Here's how the part is built. I have some questions about the finished solid (model axes, mm). A direction names the side the tool comes from. Round coordinates to 2 decimals unless told otherwise and drop trailing zeros. Write each loop counter-clockwise with the first axis right and the second up, starting at its lowest first coordinate (ties: lowest second). Pieces come first, ordered by that corner, then holes. Notation, with made-up numbers: (54, 54) -> (110, 54) arc R9 ccw to (110, 64) -> close; hole circle Ø6 at (-20, -30). An arc over 180 degrees is marked (long way). Answer in a Markdown table with one row per item. Add a question column.
from build123d import *

# Parameters (mm, degrees)
SKETCH1_W           = 110
SKETCH1_H           = 40
BOSS_EXTRUDE1_DEPTH = 3
SKETCH2_W           = 2.62
SKETCH2_H           = 5
SKETCH2_R           = 4.9365
SKETCH2_R_2         = 1.125
SKETCH2_R_3         = 5.435
CUT_EXTRUDE1_DEPTH  = 4


with BuildPart() as part:
    # Sketch1 → Boss-Extrude1 (new body)
    with BuildSketch(Plane.XY):
        with Locations((55, 20)):
            Rectangle(SKETCH1_W, SKETCH1_H)
    extrude(amount=BOSS_EXTRUDE1_DEPTH)

    # Sketch2 → Cut-Extrude1 (cut, through all)
    with BuildSketch(Plane.XY.offset(3)):
        with Locations((98.94, 37.5)):
            Rectangle(SKETCH2_W, SKETCH2_H)
        with Locations((75.06, 37.5)):
            Rectangle(SKETCH2_W, SKETCH2_H)
        with Locations((75.06, 27.5)):
            Rectangle(SKETCH2_W, SKETCH2_H)
        with Locations((75.06, 17.5)):
            Rectangle(SKETCH2_W, SKETCH2_H)
        with Locations((75.06, 7.5)):
            Rectangle(SKETCH2_W, SKETCH2_H)
        with Locations((98.94, 27.5)):
            Rectangle(SKETCH2_W, SKETCH2_H)
        with Locations((98.94, 17.5)):
            Rectangle(SKETCH2_W, SKETCH2_H)
        with Locations((98.94, 7.5)):
            Rectangle(SKETCH2_W, SKETCH2_H)
        with Locations((33, 20)):
            Circle(SKETCH2_R)
        with Locations((57, 20)):
            Circle(SKETCH2_R)
        with Locations((2.5, 37.5)):
            Circle(SKETCH2_R_2)
        with Locations((107.5, 37.5)):
            Circle(SKETCH2_R_2)
        with Locations((107.5, 2.5)):
            Circle(SKETCH2_R_2)
        with Locations((2.5, 2.5)):
            Circle(SKETCH2_R_2)
        with Locations((87, 20)):
            Circle(SKETCH2_R_3)
    extrude(amount=-CUT_EXTRUDE1_DEPTH, mode=Mode.SUBTRACT)


solid = part.part
Item 1: If we mould it in two halves opening along Y, with no side actions, what happens to faces 1 (the flat face through (73.75, 7, 2)), 2 (the flat face through (54, 0, 1)), 3 (the flat face through (100.25, 37, 2)), 4 (the flat face through (76.37, 7, 2))? For each: pulls with the +Y half, pulls with the -Y half, needs draft (parallel to the pull), parting line crosses it, or undercut.
Item 2: If we section it at B-B on x = 87: Please give me the cut outline in (y, z) (3 decimals).
Item 3: If we section it at C-C on y = 2.5: Please give me the cut outline in (x, z) (3 decimals), then the cut area to 4 significant figures.
Item 4: I need wall thicknesses on line 1 along Y through (x, z) = (2.5, 0.85) (3 decimals); line 2 along X through (y, z) = (9, 1.7); line 3 along X through (y, z) = (21.5, 2.65). Which ranges of each line are inside material? Lowest first, please. Write a range as from..to.
Item 5: For P1, Ø1.3, axis at x = 75, z = 1.5, coming from the +Y side; P2, Ø1.3, axis at x = 99.5, z = 1.5, coming from the -Y side; P3, Ø8, axis at x = 57, y = 20, coming from the -Z side, each with a flat end and sliding along its axis, tell me the tip position at first contact or that it passes through.
Item 6: On a 3-axis mill with a long thin cutter (end or side, diameter ignored), from which of +Z, -Z, +X, -X, +Y, -Y can I reach the whole of each face in a straight line? I mean faces 5 (the flat face through (100.25, 27, 2)), 6 (the flat face through (87, 40, 1)), 7 (the flat face through (97.63, 37, 2)). Say none if no direction works.
Item 7: If we section it at D-D on z = 2.3: Give the number of separate pieces and of enclosed holes in the cut face, then the cut area to 3 significant figures.
Item 8: If we section it at A-A on x = 2.5: Please give me the cut outline in (y, z) (3 decimals).
Results list:
| question | item | result |
|---|---|---|
| 1 | face 1 | undercut |
| 1 | face 2 | pulls with the -Y half |
| 1 | face 3 | needs draft |
| 1 | face 4 | undercut |
| 2 | outline | (0, 0) -> (14.565, 0) -> (14.565, 3) -> (0, 3) -> close; (25.435, 0) -> (40, 0) -> (40, 3) -> (25.435, 3) -> close |
| 3 | outline | (0, 0) -> (1.375, 0) -> (1.375, 3) -> (0, 3) -> close; (3.625, 0) -> (106.375, 0) -> (106.375, 3) -> (3.625, 3) -> close; (108.625, 0) -> (110, 0) -> (110, 3) -> (108.625, 3) -> close |
| 3 | area | 316.5 mm² |
| 4 | line 1 | 0..1.375, 3.625..36.375, 38.625..40 |
| 4 | line 2 | 0..73.75, 76.37..97.63, 100.25..110 |
| 4 | line 3 | 0..28.3, 37.7..52.3, 61.7..81.78, 92.22..110 |
| 5 | P1 | y = 35 |
| 5 | P2 | y = 0 |
| 5 | P3 | through |
| 6 | face 5 | +Z, -Z |
| 6 | face 6 | +Z, -Z, +X, -X, +Y |
| 6 | face 7 | +Z, -Z, +Y |
| 7 | separate pieces | 1 |
| 7 | enclosed holes | 13 |
| 7 | area | 4,030 mm² |
| 8 | outline | (0, 0) -> (1.375, 0) -> (1.375, 3) -> (0, 3) -> close; (3.625, 0) -> (36.375, 0) -> (36.375, 3) -> (3.625, 3) -> close; (38.625, 0) -> (40, 0) -> (40, 3) -> (38.625, 3) -> close |
